Model file for the job. Use its own axes, mm. Coordinates: 2 decimals unless noted, no trailing zeros. Write each loop counter-clockwise with the first axis right and the second up, starting at its lowest first coordinate (ties: lowest second). Pieces come first, ordered by that corner, then holes. Notation, with made-up numbers: (69, 24) -> (80, 24) arc R21 ccw to (80, 46) -> close; hole circle Ø9 at (-20.5, -6). An arc over 180 degrees is marked (long way). Write item = value, one per line. Start each with the question number.
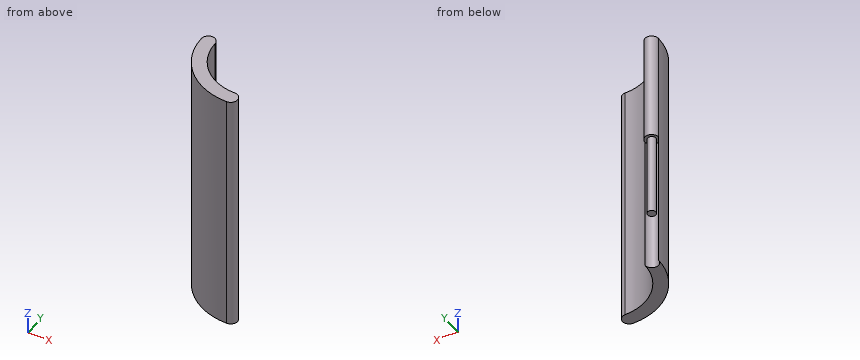
from build123d import *

# Parameters (mm, degrees)
BOSS_EXTRU_1_DEPTH = 450
ESQUISSE1_3_R      = 7.5
BOSS_EXTRU_2_DEPTH = 350
ESQUISSE1_4_R      = 12.5
ESQUISSE1_4_R_2    = 7.5
BOSS_EXTRU_3_DEPTH = 200


with BuildPart() as part:
    # Esquisse1 → Boss.-Extru.1 (new body)
    with BuildSketch(Plane.XY):
        with BuildLine():
            ThreePointArc((-6e-09, -89), (-62.932503528, -62.932503523), (-89, 0))
            ThreePointArc((-89, 0), (-101.500000043, -12.5), (-114, 8.5e-08))
            ThreePointArc((-114, 8.5e-08), (-80.610173059, -80.610173051), (7.4e-08, -114))
            ThreePointArc((7.4e-08, -114), (12.5, -101.49999996), (-6e-09, -89))
        make_face()
    extrude(amount=-BOSS_EXTRU_1_DEPTH)



with BuildPart() as body_2:
    # Esquisse1_3 → Boss.-Extru.2 (new body)
    with BuildSketch(Plane.XY):
        with Locations((-101.5, 0)):
            Circle(ESQUISSE1_3_R)
    extrude(amount=-BOSS_EXTRU_2_DEPTH)


with BuildPart() as part_1:
    add(part.part)

    add(body_2.part)  # Boss.-Extru.3 merges body 2
    # Esquisse1_4 → Boss.-Extru.3 (add)
    with BuildSketch(Plane.XY):
        with Locations((-101.5, 0)):
            Circle(ESQUISSE1_4_R)
        with Locations((-101.5, 0)):
            Circle(ESQUISSE1_4_R_2, mode=Mode.SUBTRACT)
    extrude(amount=-BOSS_EXTRU_3_DEPTH)


solid = part_1.part
(1) Saw through at B-B (x = -101.5). Give the cut face in (y, z).
(2) Drill centre lines: line 1 along Y through (x, z) = (-3, -292.5); line 2 along X through (y, z) = (-1, -164); line 3 along X through (y, z) = (-19, -326). Where is each one in solid material? Low to high.
(3) Saw through at D-D (z = -30.5). Give the cut face in (x, y), then the cut area to 3 significant figures.
(4) Saw through at C-C (y = -101.5). Give the cut face in (x, z).
(5) Drop flat-ended pins along their axis: pin 1 Ø5 at (y, z) = (-92, -404.5) entering from +X; pin 2 Ø4 at (y, z) = (-21, -186.5) entering from +X; pin 3 Ø10 at (x, z) = (-58.5, -203.5) entering from +Y; pin 4 Ø8 at (x, y) = (-81, -3) entering from +Z. Give the stop position or say it passes through.
(6) Saw through at A-A (z = -216.5). Give the cut face in (x, y), then the cut area to 3 significant figures.
Returned:
q1.outline = (-51.9, -450) -> (-12.5, -450) -> (-12.5, -200) -> (-7.5, -200) -> (-7.5, -350) -> (7.5, -350) -> (7.5, -200) -> (12.5, -200) -> (12.5, 0) -> (-51.9, 0) -> close
q2.line_1 = -113.96 to -88.95
q2.line_2 = -114 to -88.99
q2.line_3 = -112.41 to -86.95
q3.outline = (-114, 0) arc R114 ccw to (0, -114) arc R12.5 ccw to (0, -89) arc R89 cw to (-89, 0) arc R12.5 ccw to start
q3.area = 4,480 mm2
q4.outline = (-51.9, -450) -> (12.5, -450) -> (12.5, 0) -> (-51.9, 0) -> close
q5.pin_1 = 10.36
q5.pin_2 = -85.98
q5.pin_3 = -62.36
q5.pin_4 = through
q6.outline = (-114, 0) arc R114 ccw to (0, -114) arc R12.5 ccw to (0, -89) arc R89 cw to (-89, 0) arc R12.5 cw to start; circle Ø15 at (-101.5, 0)
q6.area = 4,160 mm2
